Geometry check sheet. Reference: the model listing, model coordinates, mm. Face numbers are marked on the shaded views. Give positions to 0.01 mm unless a question says otherwise; leave off trailing zeros. Loops run counter-clockwise (first coordinate to the right, second up) from the corner with the lowest first, then second, coordinate; pieces in that order, holes last. Notation, with made-up numbers: (68, -10) -> (127, -10) arc R16 ccw to (127, 21) -> close; hole circle Ø3 at (85.5, 29). An arc over 180 degrees is marked (long way). Write item = value, one per line.
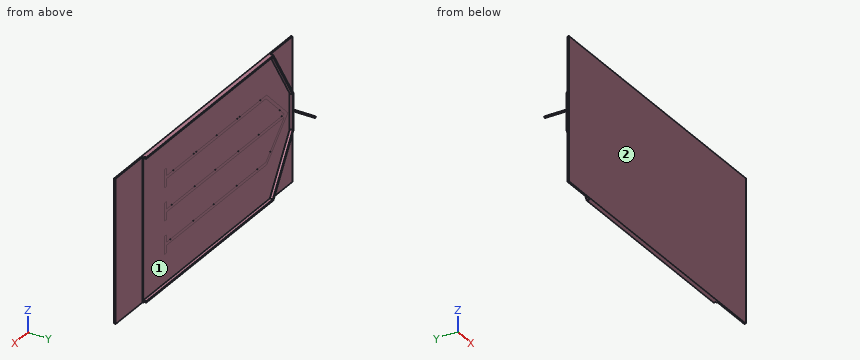
```python
from build123d import *

# Parameters (mm, degrees)
SKETCH1_W             = 2438.4
SKETCH1_H             = 1219.2
BASE_DEPTH            = 12.7
OUTSIDE_WALLS_DEPTH   = 25.4
SKETCH3_W             = 12.7
SKETCH3_H             = 1219.2
FRONT_WALL_DEPTH      = 6.35
TAPE_DEPTH            = 0.1
SKETCH5_R             = 6.35
F_10KHZ_EMITTER_DEPTH = 203.2


with BuildPart() as part:
    # Sketch1 → Base (new body)
    with BuildSketch(Plane(origin=(0, 0, 0), x_dir=(1, 0, 0), z_dir=(0, 1, 0))):
        with Locations((1219.2, -609.6)):
            Rectangle(SKETCH1_W, SKETCH1_H)
    extrude(amount=BASE_DEPTH)

    # Sketch2 → Outside Walls (add)
    with BuildSketch(Plane(origin=(0, 12.7, 0), x_dir=(1, 0, 0), z_dir=(0, 1, 0))):
        Polygon((304.8, 0), (25.4, -457.2), (25.4, -762), (304.8, -1219.2), (2057.4, -1219.2), (2057.4, -1206.5), (311.922599639, -1206.5), (38.1, -758.426655137), (38.1, -460.773344863), (311.922599639, -12.7), (2057.4, -12.7), (2057.4, 0), align=None)
    extrude(amount=OUTSIDE_WALLS_DEPTH)

    # Sketch3 → Front Wall (add)
    with BuildSketch(Plane(origin=(0, 12.7, 0), x_dir=(1, 0, 0), z_dir=(0, 1, 0))):
        with Locations((2063.75, -609.6)):
            Rectangle(SKETCH3_W, SKETCH3_H)
    extrude(amount=FRONT_WALL_DEPTH)

    # Sketch4 → Tape (add)
    with BuildSketch(Plane(origin=(0, 12.7, 0), x_dir=(1, 0, 0), z_dir=(0, 1, 0))):
        Polygon((63.5, -609.6), (355.6, -901.7), (1739.9, -901.7), (1739.9, -965.2), (1765.3, -965.2), (1765.3, -812.8), (1739.9, -812.8), (1739.9, -876.3), (366.121024484, -876.3), (112.121024484, -622.3), (1739.9, -622.3), (1739.9, -685.8), (1765.3, -685.8), (1765.3, -533.4), (1739.9, -533.4), (1739.9, -596.9), (112.121024484, -596.9), (366.121024484, -342.9), (1739.9, -342.9), (1739.9, -406.4), (1765.3, -406.4), (1765.3, -254), (1739.9, -254), (1739.9, -317.5), (355.6, -317.5), align=None)
    extrude(amount=TAPE_DEPTH)

    # Sketch5 → 10kHz Emitter (add)
    with BuildSketch(Plane(origin=(0, 12.7, 0), x_dir=(1, 0, 0), z_dir=(0, 1, 0))):
        with Locations((12.7, -609.6)):
            Circle(SKETCH5_R)
    extrude(amount=F_10KHZ_EMITTER_DEPTH)


solid = part.part
```
Item 1: Section check A-A, the plane x = 462. Record the cut outline in (y, z).
Answer:
outline = (0, 0) -> (38.1, 0) -> (38.1, 12.7) -> (12.7, 12.7) -> (12.7, 317.5) -> (12.8, 317.5) -> (12.8, 342.9) -> (12.7, 342.9) -> (12.7, 596.9) -> (12.8, 596.9) -> (12.8, 622.3) -> (12.7, 622.3) -> (12.7, 876.3) -> (12.8, 876.3) -> (12.8, 901.7) -> (12.7, 901.7) -> (12.7, 1206.5) -> (38.1, 1206.5) -> (38.1, 1219.2) -> (0, 1219.2) -> close
Item 2: Thickness scan on L1, parallel to Z at x = 1129.5, y = 29.5; L2, parallel to Y at x = 1132, z = 967; L3, parallel to X at y = 15, z = 400. Record the ranges inside material, lowest first. Write a range as [from, to].
Answer:
L1 = [0, 12.7], [1206.5, 1219.2]
L2 = [0, 12.7]
L3 = [60.36, 75.24], [2057.4, 2070.1]
Item 3: Gauge pin test, flat ends, axial feed: pin 1 (14 mm diameter, centred on x = 2063, z = 754.5, fed in from +Y); pin 2 (1.5 mm diameter, centred on x = 1556, z = 991.5, fed in from +Y); pin 3 (7 mm diameter, centred on y = 15, z = 406, fed in from -X); pin 4 (10 mm diameter, centred on y = 27.5, z = 1214.5, fed in from +X). Record the tip position at first contact, or that the pin passes through.
Answer:
pin_1 = 19.05
pin_2 = 12.7
pin_3 = 0
pin_4 = 2057.4
Item 4: Section check C-C, the plane y = 110. Record the cut outline in (x, z).
Answer:
outline = circle Ø12.7 at (12.7, 609.6)
Item 5: Draft check along Z on the marked faces 1 and 2. Enter one of: +Z half, -Z half, draft (parallel to the pull), parting line (faces both ways), or undercut.
Answer:
face_1 = undercut
face_2 = draft
Item 6: Section check D-D, the plane z = 1120. Record the cut outline in (x, y).
Answer:
outline = (0, 0) -> (2438.4, 0) -> (2438.4, 12.7) -> (2070.1, 12.7) -> (2070.1, 19.05) -> (2057.4, 19.05) -> (2057.4, 12.7) -> (259.06, 12.7) -> (259.06, 38.1) -> (244.18, 38.1) -> (244.18, 12.7) -> (0, 12.7) -> close
Item 7: Section check B-B, the plane z = 731.5. Record the cut outline in (x, y).
Answer:
outline = (0, 0) -> (2438.4, 0) -> (2438.4, 12.7) -> (2070.1, 12.7) -> (2070.1, 19.05) -> (2057.4, 19.05) -> (2057.4, 12.7) -> (221.32, 12.7) -> (221.32, 12.8) -> (185.4, 12.8) -> (185.4, 12.7) -> (38.1, 12.7) -> (38.1, 38.1) -> (25.4, 38.1) -> (25.4, 12.7) -> (0, 12.7) -> close
